Can you work these out from the model? Positions are in its coordinate system, mm. Coordinates: 2 decimals unless noted, no trailing zeros. Loops run counter-clockwise (first coordinate to the right, second up) from the corner with the lowest first, then second, coordinate; pieces in that order, holes last. Notation, with made-up numbers: (-33, 39.5) - (-16, 39.5) arc R34 ccw to (-16, 76.5) - close; hole circle Ø9 at (-35.5, 21). An arc over 180 degrees is marked (long way). Put each result on its own line as item: value. Start each with the question number.
from build123d import *

# Parameters (mm, degrees)
SKETCH1_W           = 160
SKETCH1_H           = 100
BOSS_EXTRUDE1_DEPTH = 4.5
FILLET1_R           = 10
SKETCH2_W           = 4.5
SKETCH2_H           = 20
CUT_EXTRUDE1_DEPTH  = 5
SKETCH3_W           = 50
SKETCH3_H           = 30
BOSS_EXTRUDE2_DEPTH = 4.5
FILLET2_R           = 5
SKETCH4_W           = 4.5
SKETCH4_H           = 2.5
SKETCH4_W_2         = 2.5
SKETCH4_H_2         = 4.5
CUT_EXTRUDE2_DEPTH  = 4.5


with BuildPart() as part:
    # Sketch1 → Boss-Extrude1 (new body)
    with BuildSketch(Plane.XY):
        Rectangle(SKETCH1_W, SKETCH1_H)
    extrude(amount=BOSS_EXTRUDE1_DEPTH)

    # Fillet1
    fillet1_edges = [part.edges().sort_by_distance(p)[0] for p in [
        (80, -50, 2.25),
        (-80, -50, 2.25),
        (-80, 50, 2.25),
        (80, 50, 2.25),
    ]]
    fillet(fillet1_edges, radius=FILLET1_R)

    # Sketch2 → Cut-Extrude1 (cut)
    with BuildSketch(Plane.XY.offset(4.5)):
        with Locations((-59.45, 25)):
            Rectangle(SKETCH2_W, SKETCH2_H)
        with Locations((-59.45, -25)):
            Rectangle(SKETCH2_W, SKETCH2_H)
        with Locations((59.45, -25)):
            Rectangle(SKETCH2_W, SKETCH2_H)
        with Locations((59.45, 25)):
            Rectangle(SKETCH2_W, SKETCH2_H)
    extrude(amount=-CUT_EXTRUDE1_DEPTH, mode=Mode.SUBTRACT)

    # Sketch3 → Boss-Extrude2 (add)
    with BuildSketch(Plane.XY.offset(4.5)):
        with Locations((0, 65)):
            Rectangle(SKETCH3_W, SKETCH3_H)
    extrude(amount=-BOSS_EXTRUDE2_DEPTH)

    # Fillet2
    fillet2_edges = [part.edges().sort_by_distance(p)[0] for p in [
        (-25, 80, 2.25),
        (25, 80, 2.25),
    ]]
    fillet(fillet2_edges, radius=FILLET2_R)

    # Sketch4 → Cut-Extrude2 (cut)
    with BuildSketch(Plane.XY.offset(4.5)):
        with Locations((0, 78.75)):
            Rectangle(SKETCH4_W, SKETCH4_H)
        with Locations((26.25, 62.5)):
            Rectangle(SKETCH4_W_2, SKETCH4_H_2)
        with Locations((23.75, 62.5)):
            Rectangle(SKETCH4_W_2, SKETCH4_H_2)
        with Locations((-23.75, 62.5)):
            Rectangle(SKETCH4_W_2, SKETCH4_H_2)
        with Locations((0, 46.25)):
            Rectangle(SKETCH4_W, SKETCH4_H)
    extrude(amount=-CUT_EXTRUDE2_DEPTH, mode=Mode.SUBTRACT)


solid = part.part
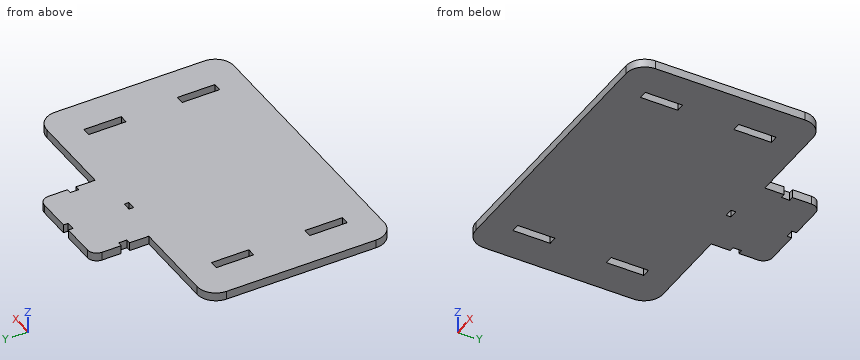
Q1. Will these pins go through, and if not, where does the flat tip stop? pin 1 (2 mm diameter, centred on y = 65, z = 2.5, fed in from -X); pin 2 (0.8 mm diameter, centred on y = 47, z = 2.5, fed in from -X); pin 3 (2 mm diameter, centred on y = 55.5, z = 3, fed in from +X).
Q2. I want a section at C-C on x = -45. List the corners of the cut face in (y, z) for me, and give its area (3 significant figures).
Q3. I want a section at A-A on x = 0. List the corners of the cut face in (y, z) for me, and give its area (4 significant figures).
Q4. I want a section at D-D on y = 72.5. List the corners of the cut face in (x, z) for me, and give its area (3 significant figures).
Q5. Please list where these lines run through material, in increasing order: line 1 along X through (y, z) = (31, 1.55); line 2 along Y through (x, z) = (-43, 2.1); line 3 along X through (y, z) = (59, 3.3). Write a range as [from, to].
Q6. I want a section at B-B on z = 1.5. Count the separate pieces of the cut face and the enclosed holes in it, and give its area (3 significant figures).
Calculated:
1. pin 1: x = -25
1. pin 2: x = -77.51
1. pin 3: x = 25
2. outline: (-50, 0) - (50, 0) - (50, 4.5) - (-50, 4.5) - close
2. area: 450 mm2
3. outline: (-50, 0) - (45, 0) - (45, 4.5) - (-50, 4.5) - close; (47.5, 0) - (77.5, 0) - (77.5, 4.5) - (47.5, 4.5) - close
3. area: 562.5 mm2
4. outline: (-25, 0) - (25, 0) - (25, 4.5) - (-25, 4.5) - close
4. area: 225 mm2
5. line 1: [-80, -61.7], [-57.2, 57.2], [61.7, 80]
5. line 2: [-50, 50]
5. line 3: [-25, 25]
6. separate pieces: 1
6. enclosed holes: 5
6. area: 17,000 mm2
